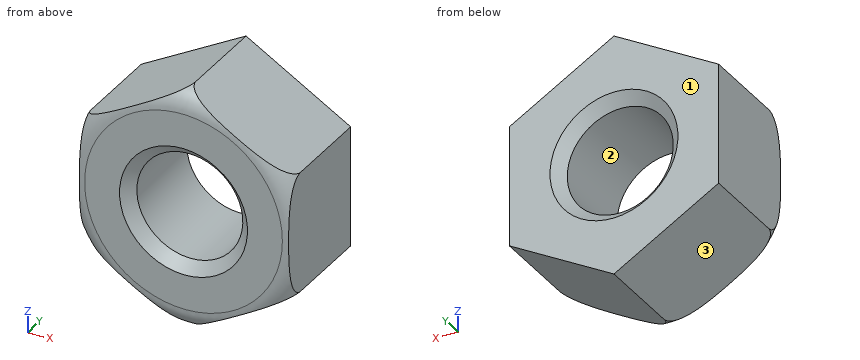
Solid Edge part; units mm, degrees
sketch "Sketch1" plane through (0, 0, 0) normal (0, -1, 0) x (1, 0, 0)
  circle A0 centre (0, 0) radius 22
extrude "Protrusion1" add sketch "Sketch1" against normal blind 19.8
fillet "Round_1" radius 4 1 edges at (-22, 0, 0)
sketch "Sketch2" plane through (0, 0, 0) normal (0, -1, 0) x (1, 0, 0)
  line L0 (0, 22) -> (-19.0525, 11)
extrude "ExtrudedCutout_1" cut sketch "Sketch2" against normal blind 127.8388 material side at (-9.5513, 0, 16.5433)
pattern_circular "Pattern1" count 6 over 360 about axis through (0, 0, 0) along (0, -1, 0) of "ExtrudedCutout_1"
hole "Hole_1" at (0, 0, 0) direction (0, 1, 0) diameter 19.294 end up to next
chamfer "Chamfer_1" distance 2 angle 45 2 edges at (-9.647, 0, 0) (0, 19.8, -9.647)
Geometry: final body of the model. Coordinates: model frame, mm. Face numbers are marked on the shaded views. Coordinates: 2 decimals unless noted, no trailing zeros. Loops run counter-clockwise (first coordinate to the right, second up) from the corner with the lowest first, then second, coordinate; pieces in that order, holes last. Notation, with made-up numbers: (7, 57.5) -> (12, 57.5) arc R3 cw to (12, 61.5) -> close; hole circle Ø4 at (61.5, -18.75). An arc over 180 degrees is marked (long way). Use a Markdown table: item, result. Add a question column.
(1) Line query: line 1 along Z through (x, y) = (0, 9); line 2 along X through (y, z) = (12, 0); line 3 along Z through (x, y) = (1.5, 18.25). Output: solid intervals per line, ascending.
(2) Section query B-B, the plane z = 0. Return loops of the section in (x, y).
(3) Section query A-A, the plane y = 15.75. Return loops of the section in (x, z), plus the area to 3 significant figures.
(4) Pin query (flat end, axial travel): pin 1 Ø6 at (x, y) = (-6.5, 14.5) entering from -Z; pin 2 Ø4 at (x, z) = (-9, -2.5) entering from +Y; pin 3 Ø1.5 at (y, z) = (2, -10) entering from -X; pin 4 Ø1.5 at (x, y) = (-15, 17) entering from +Z. Return the tip coordinate at first contact, or that it passes through.
(5) Mould query, pull axis Z, two halves, no side actions, for the marked faces 1, 2 and 3. Classes: pulls with the +Z half, pulls with the -Z half, needs draft (parallel to the pull), parting line crosses it, or undercut.
Answer:
| question | item | result |
|---|---|---|
| 1 | line 1 | z = -22 to -9.65, 9.65 to 22 |
| 1 | line 2 | x = -19.05 to -9.65, 9.65 to 19.05 |
| 1 | line 3 | z = -21.13 to -9.98, 9.98 to 21.13 |
| 2 | outline | (-19.05, 0.14) arc R4 ccw to (-18, 0) -> (-11.65, 0) -> (-9.65, 2) -> (-9.65, 17.8) -> (-11.65, 19.8) -> (-19.05, 19.8) -> close; (9.65, 2) -> (11.65, 0) -> (18, 0) arc R4 ccw to (19.05, 0.14) -> (19.05, 19.8) -> (11.65, 19.8) -> (9.65, 17.8) -> close |
| 3 | outline | (-19.05, -11) -> (0, -22) -> (19.05, -11) -> (19.05, 11) -> (0, 22) -> (-19.05, 11) -> close; hole circle Ø19.29 at (0, 0) |
| 3 | area | 965 mm^2 |
| 4 | pin 1 | stops at z = -19.98 |
| 4 | pin 2 | stops at y = 19.49 |
| 4 | pin 3 | stops at x = -19.05 |
| 4 | pin 4 | stops at z = 13.77 |
| 5 | face 1 | needs draft |
| 5 | face 2 | undercut |
| 5 | face 3 | pulls with the -Z half |
